from build123d import *

# Parameters (mm, degrees)
BOSS_EXTRUDE1_DEPTH = 40
CUT_EXTRUDE1_REACH  = 57.333
SKETCH2_R           = 2.665
CUT_EXTRUDE2_REACH  = 59.037
SKETCH3_R           = 2.665
FILLET1_R           = 2.54


with BuildPart() as part:
    # Sketch1 → Boss-Extrude1 (new body)
    with BuildSketch(Plane(origin=(0, 0, 0), x_dir=(1, 0, 0), z_dir=(0, 1, 0))):
        Polygon((0, 0), (-25.4, 0), (-25.4, 3.175), (-3.175, 3.175), (-3.175, 31.75), (0, 31.75), align=None)
    extrude(amount=BOSS_EXTRUDE1_DEPTH)

    # Sketch2 → Cut-Extrude1 (cut, up to next)
    with BuildSketch(Plane(origin=(0, 0, -3.175), x_dir=(-1, 0, 0), z_dir=(0, 0, -1)), mode=Mode.PRIVATE) as cut_extrude1_sk1:
        with Locations((14.2875, 30)):
            Circle(SKETCH2_R)
    cut_extrude1_tool1 = extrude(cut_extrude1_sk1.sketch, amount=-CUT_EXTRUDE1_REACH, mode=Mode.PRIVATE) & part.part
    # Sketch2 → Cut-Extrude1 (cut, up to next)
    with BuildSketch(Plane(origin=(0, 0, -3.175), x_dir=(-1, 0, 0), z_dir=(0, 0, -1)), mode=Mode.PRIVATE) as cut_extrude1_sk2:
        with Locations((14.2875, 10)):
            Circle(SKETCH2_R)
    cut_extrude1_tool2 = extrude(cut_extrude1_sk2.sketch, amount=-CUT_EXTRUDE1_REACH, mode=Mode.PRIVATE) & part.part
    add(cut_extrude1_tool1.solids().sort_by_distance((-14.2875, 30, -3.175))[0], mode=Mode.SUBTRACT)
    add(cut_extrude1_tool2.solids().sort_by_distance((-14.2875, 10, -3.175))[0], mode=Mode.SUBTRACT)

    # Sketch3 → Cut-Extrude2 (cut, up to next)
    with BuildSketch(Plane(origin=(0, 0, 0), x_dir=(0, 0, -1), z_dir=(1, 0, 0)), mode=Mode.PRIVATE) as cut_extrude2_sk1:
        with Locations((28.17625, 10)):
            Circle(SKETCH3_R)
    cut_extrude2_tool1 = extrude(cut_extrude2_sk1.sketch, amount=-CUT_EXTRUDE2_REACH, mode=Mode.PRIVATE) & part.part
    # Sketch3 → Cut-Extrude2 (cut, up to next)
    with BuildSketch(Plane(origin=(0, 0, 0), x_dir=(0, 0, -1), z_dir=(1, 0, 0)), mode=Mode.PRIVATE) as cut_extrude2_sk2:
        with Locations((28.17625, 30)):
            Circle(SKETCH3_R)
    cut_extrude2_tool2 = extrude(cut_extrude2_sk2.sketch, amount=-CUT_EXTRUDE2_REACH, mode=Mode.PRIVATE) & part.part
    add(cut_extrude2_tool1.solids().sort_by_distance((0, 10, -28.17625))[0], mode=Mode.SUBTRACT)
    add(cut_extrude2_tool2.solids().sort_by_distance((0, 30, -28.17625))[0], mode=Mode.SUBTRACT)

    # Fillet1
    fillet1_edges = [part.edges().sort_by_distance(p)[0] for p in [
        (-25.4, 40, -1.5875),
        (-25.4, 0, -1.5875),
        (-1.5875, 40, -31.75),
        (-1.5875, 0, -31.75),
    ]]
    fillet(fillet1_edges, radius=FILLET1_R)


solid = part.part
Part model, mm, in its own coordinate system. A direction names the side the tool comes from. Give positions to 0.01 mm unless a question says otherwise; leave off trailing zeros. Write each loop counter-clockwise with the first axis right and the second up, starting at its lowest first coordinate (ties: lowest second). Pieces come first, ordered by that corner, then holes.
1) Probe L1, parallel to Y at x = -1, z = -27; L2, parallel to X at y = 35.5, z = -10.5 (3 decimals). List the from-to ranges inside material, lowest first.
Resolved:
L1: y = 0 to 7.61, 12.39 to 27.61, 32.39 to 40
L2: x = -3.175 to 0
2) Two-plate mould, pull along Y, no slides. Class faces 3 (the face through (-1.565, 12.247, -29.609)), 4 (the face through (-1.565, 39.276, -30.986)), 5 (the face through (-24.636, 0.724, -1.61)): released by +Y, released by -Y, zero draft, split by the parting line, or undercut.
Resolved:
face 3: undercut
face 4: released by +Y
face 5: released by -Y
3) Cut at B-B on x = -16.25. Write the cut outline in (y, z) (3 decimals).
Resolved:
outline: (0, -3.175) - (8.197, -3.175) - (8.197, 0) - (0, 0) - close; (11.803, -3.175) - (28.197, -3.175) - (28.197, 0) - (11.803, 0) - close; (31.803, -3.175) - (40, -3.175) - (40, 0) - (31.803, 0) - close
4) Pin check, flat tips, straight feed: pin 1 (12 mm diameter, centred on x = -13, z = -20.5, fed in from +Y); pin 2 (6.5 mm diameter, centred on x = -17.5, y = 21, fed in from -Z) (3 decimals); pin 3 (1.5 mm diameter, centred on y = 29.5, z = -25.5, fed in from -X) (3 decimals). Stop position of each tip, or through.
Resolved:
pin 1: passes through
pin 2: stops at z = -3.175
pin 3: stops at x = -3.175
5) Cut at A-A on y = 30. State how many separate pieces and enclosed holes the cut face has, then the cut area to 3 significant figures.
Resolved:
separate pieces: 3
enclosed holes: 0
area: 138 mm2
6) Cut at C-C on z = -10. Write the cut outline in (x, y) (3 decimals), then the cut area to 3 significant figures.
Resolved:
outline: (-3.175, 0) - (0, 0) - (0, 40) - (-3.175, 40) - close
area: 127 mm2
7) Which spindle directions (+Z, -Z, +X, -X, +Y, -Y) get a long thin tool onto all of the face, cutting with end or side? Do faces 1 (the face through (-3.175, 20, -17)), 2 (the face through (-1.565, 0.724, -30.986)). Say none if no direction does.
Resolved:
face 1: -Z, -X, +Y, -Y
face 2: -Z, +X, -X, -Y
8) Cut at D-D on y = 9.5. Write the cut outline in (x, z) (3 decimals), then the cut area to 3 significant figures.
Resolved:
outline: (-25.4, -3.175) - (-16.905, -3.175) - (-16.905, 0) - (-25.4, 0) - close; (-11.67, -3.175) - (-3.175, -3.175) - (-3.175, -25.559) - (0, -25.559) - (0, 0) - (-11.67, 0) - close; (-3.175, -31.75) - (0, -31.75) - (0, -30.794) - (-3.175, -30.794) - close
area: 138 mm2
